Can you work these out from the model? Positions are in its coordinate system, mm. Coordinates: 2 decimals unless noted, no trailing zeros. Write each loop counter-clockwise with the first axis right and the second up, starting at its lowest first coordinate (ties: lowest second). Pieces come first, ordered by that corner, then holes. Notation, with made-up numbers: (-11, -29.5) -> (47, -29.5) arc R8 cw to (47, -17.5) -> close; hole circle Ø4 at (44.25, 72). An arc over 180 degrees is marked (long way). Use one line per item in the form item = value.
Autodesk Inventor part; units mm, degrees
ref_plane "YZ Plane" through (0, 0, 0) normal (1, 0, 0) x (0, 1, 0)
ref_plane "XZ Plane" through (0, 0, 0) normal (0, 1, 0) x (-1, 0, 0)
ref_plane "XY Plane" through (0, 0, 0) normal (0, 0, 1) x (1, 0, 0)
sketch "Sketch3" plane through (0, 0, 0) normal (0, 1, 0) x (-1, 0, 0)
  line L0 (-27.5, -27.5) -> (27.5, -27.5) construction
  line L1 (27.5, -27.5) -> (27.5, 27.5) construction
  line L2 (27.5, 27.5) -> (-27.5, 27.5) construction
  line L3 (-27.5, 27.5) -> (-27.5, -27.5) construction
  line L4 (-27.5, -27.5) -> (27.5, 27.5) construction
  line L5 (27.5, -27.5) -> (-27.5, 27.5) construction
  circle A0 centre (-27.5, 27.5) radius 1.6
  circle A1 centre (27.5, 27.5) radius 1.6
  circle A2 centre (-27.5, -27.5) radius 1.6
  circle A3 centre (27.5, -27.5) radius 1.6
  circle A4 centre (-67.1751, -42.4264) radius 1.6 construction
  line L6 (-27.5, -27.5) -> (-67.1751, -42.4264) construction
  line L7 (-30, -25.7695) -> (-68.0554, -40.0865) construction
  line L8 (-66.2948, -44.7663) -> (-27.0453, -30) construction
  arc A5 (-68.0554, -40.0865) -> (-66.2948, -44.7663) centre (-67.1751, -42.4264) ccw construction
  circle A6 centre (67.1751, -42.4264) radius 1.6 construction
  line L9 (27.5, -27.5) -> (67.1751, -42.4264) construction
  line L10 (27.0453, -30) -> (66.2948, -44.7663) construction
  line L11 (68.0554, -40.0865) -> (30, -25.7695) construction
  arc A7 (66.2948, -44.7663) -> (68.0554, -40.0865) centre (67.1751, -42.4264) ccw construction
  line L12 (27.5, -27.5) -> (-27.5, -27.5) construction
  line L13 (25, -25) -> (-25, -25) construction
  line L14 (-27.0453, -30) -> (27.0453, -30) construction
  line L15 (-27.5, -27.5) -> (-27.5, 27.5) construction
  line L16 (-25, -25) -> (-25, 25) construction
  line L17 (-30, 25.7695) -> (-30, -25.7695) construction
  circle A8 centre (-67.1751, 42.4264) radius 1.6 construction
  line L18 (-27.5, 27.5) -> (-67.1751, 42.4264) construction
  line L19 (-27.0453, 30) -> (-66.2948, 44.7663) construction
  line L20 (-68.0554, 40.0865) -> (-30, 25.7695) construction
  arc A9 (-66.2948, 44.7663) -> (-68.0554, 40.0865) centre (-67.1751, 42.4264) ccw construction
  line L21 (-27.5, 27.5) -> (27.5, 27.5) construction
  line L22 (-25, 25) -> (25, 25) construction
  line L23 (27.0453, 30) -> (-27.0453, 30) construction
  circle A10 centre (67.1751, 42.4264) radius 1.6 construction
  line L24 (27.5, 27.5) -> (67.1751, 42.4264) construction
  line L25 (34.5998, 27.5) -> (68.0554, 40.0865) construction
  line L26 (66.2948, 44.7663) -> (27.0453, 30) construction
  arc A11 (68.0554, 40.0865) -> (66.2948, 44.7663) centre (67.1751, 42.4264) ccw construction
  line L27 (27.5, -27.5) -> (27.5, 27.5) construction
  line L28 (30, -25.7695) -> (30, 25.7695) construction
  line L29 (25, 25) -> (25, -25) construction
  line L30 (34.5998, 27.5) -> (30, 25.7695) construction
  line L31 (55, 55) -> (-55, -55) construction
  line L32 (-55, 55) -> (55, -55) construction
  circle A12 centre (0, 0) radius 110 construction
  arc A13 (43.0581, -98.5) -> (-43.0581, -98.5) centre (0, 0) ccw construction
  line L33 (0, -107.5) -> (0, -98.5) construction
  line L34 (0, -98.5) -> (0, -73.5) construction
  line L35 (0, -98.5) -> (-43.0581, -98.5) construction
  line L36 (0, -98.5) -> (43.0581, -98.5) construction
  line L37 (43.0581, -98.5) -> (-43.0581, -98.5) construction
  line L38 (-18.0581, -73.5) -> (18.0581, -73.5) construction
  arc A14 (43.0581, -98.5) -> (18.0581, -73.5) centre (18.0581, -98.5) ccw construction
  arc A15 (-18.0581, -73.5) -> (-43.0581, -98.5) centre (-18.0581, -98.5) ccw construction
  line L39 (0, 107.5) -> (0, 97.5) construction
  line L40 (0, 97.5) -> (-22.5, 97.5) construction
  line L41 (-22.5, 97.5) -> (-22.5, 82.5) construction
  line L42 (22.5, 82.5) -> (22.5, 97.5) construction
  line L43 (22.5, 90) -> (-22.5, 90) construction
  line L44 (15, 97.5) -> (-15, 97.5)
  line L45 (-15, 82.5) -> (15, 82.5)
  arc A16 (15, 82.5) -> (15, 97.5) centre (15, 90) ccw
  arc A17 (-15, 97.5) -> (-15, 82.5) centre (-15, 90) ccw
  line L46 (22.5, 82.5) -> (17.5, 82.5) construction
  line L47 (17.5, 82.5) -> (17.5, 77.5) construction
  circle A18 centre (17.5, 77.5) radius 1.6
  circle A19 centre (-17.5, 77.5) radius 1.6
  line L48 (-58.3363, 79.5495) -> (-79.5495, 58.3363) construction
  arc A20 (-47.7297, 68.9429) -> (-58.3363, 79.5495) centre (-53.033, 74.2462) ccw construction
  arc A21 (-79.5495, 58.3363) -> (-68.9429, 47.7297) centre (-74.2462, 53.033) ccw construction
  line L49 (-68.9429, 47.7297) -> (-47.7297, 68.9429) construction
  circle A22 centre (-67.1751, 42.4264) radius 1.6 construction
  circle A23 centre (-42.4264, 67.1751) radius 1.6 construction
  line L50 (-97.5, 15) -> (-97.5, -15)
  arc A24 (-82.5, 15) -> (-97.5, 15) centre (-90, 15) ccw
  arc A25 (-97.5, -15) -> (-82.5, -15) centre (-90, -15) ccw
  line L51 (-82.5, -15) -> (-82.5, 15)
  circle A26 centre (-77.5, -17.5) radius 1.6
  circle A27 centre (-77.5, 17.5) radius 1.6
  line L52 (-79.5495, -58.3363) -> (-58.3363, -79.5495) construction
  arc A28 (-68.9429, -47.7297) -> (-79.5495, -58.3363) centre (-74.2462, -53.033) ccw construction
  arc A29 (-58.3363, -79.5495) -> (-47.7297, -68.9429) centre (-53.033, -74.2462) ccw construction
  line L53 (-47.7297, -68.9429) -> (-68.9429, -47.7297) construction
  circle A30 centre (-42.4264, -67.1751) radius 1.6 construction
  circle A31 centre (-67.1751, -42.4264) radius 1.6 construction
  line L54 (-15, -97.5) -> (15, -97.5)
  arc A32 (-15, -82.5) -> (-15, -97.5) centre (-15, -90) ccw
  arc A33 (15, -97.5) -> (15, -82.5) centre (15, -90) ccw
  line L55 (15, -82.5) -> (-15, -82.5)
  circle A34 centre (17.5, -77.5) radius 1.6
  circle A35 centre (-17.5, -77.5) radius 1.6
  line L56 (58.3363, -79.5495) -> (79.5495, -58.3363) construction
  arc A36 (47.7297, -68.9429) -> (58.3363, -79.5495) centre (53.033, -74.2462) ccw construction
  arc A37 (79.5495, -58.3363) -> (68.9429, -47.7297) centre (74.2462, -53.033) ccw construction
  line L57 (68.9429, -47.7297) -> (47.7297, -68.9429) construction
  circle A38 centre (67.1751, -42.4264) radius 1.6 construction
  circle A39 centre (42.4264, -67.1751) radius 1.6 construction
  line L58 (97.5, -15) -> (97.5, 15)
  arc A40 (82.5, -15) -> (97.5, -15) centre (90, -15) ccw
  arc A41 (97.5, 15) -> (82.5, 15) centre (90, 15) ccw
  line L59 (82.5, 15) -> (82.5, -15)
  circle A42 centre (77.5, 17.5) radius 1.6
  circle A43 centre (77.5, -17.5) radius 1.6
  line L60 (79.5495, 58.3363) -> (58.3363, 79.5495) construction
  arc A44 (68.9429, 47.7297) -> (79.5495, 58.3363) centre (74.2462, 53.033) ccw construction
  arc A45 (58.3363, 79.5495) -> (47.7297, 68.9429) centre (53.033, 74.2462) ccw construction
  line L61 (47.7297, 68.9429) -> (68.9429, 47.7297) construction
  circle A46 centre (42.4264, 67.1751) radius 1.6 construction
  circle A47 centre (67.1751, 42.4264) radius 1.6 construction
  line L62 (58.3363, -58.3363) -> (51.2652, -51.2652) construction
  line L63 (40.6586, -61.8718) -> (61.8718, -40.6586) construction
  arc A48 (40.6586, -61.8718) -> (44.5267, -89.5398) centre (53.033, -74.2462) ccw construction
  arc A49 (89.5398, -44.5267) -> (61.8718, -40.6586) centre (74.2462, -53.033) ccw construction
  line L64 (0, -73.5) -> (0, -66.5) construction
  arc A50 (44.5267, 89.5398) -> (40.6586, 61.8718) centre (53.033, 74.2462) ccw construction
  line L65 (61.8718, 40.6586) -> (40.6586, 61.8718) construction
  arc A51 (61.8718, 40.6586) -> (89.5398, 44.5267) centre (74.2462, 53.033) ccw construction
  arc A52 (-89.5398, 44.5267) -> (-61.8718, 40.6586) centre (-74.2462, 53.033) ccw construction
  line L66 (-40.6586, 61.8718) -> (-61.8718, 40.6586) construction
  arc A53 (-40.6586, 61.8718) -> (-44.5267, 89.5398) centre (-53.033, 74.2462) ccw construction
  arc A54 (-44.5267, -89.5398) -> (-40.6586, -61.8718) centre (-53.033, -74.2462) ccw construction
  line L67 (-61.8718, -40.6586) -> (-40.6586, -61.8718) construction
  arc A55 (-61.8718, -40.6586) -> (-89.5398, -44.5267) centre (-74.2462, -53.033) ccw construction
  arc A56 (89.5398, -44.5267) -> (89.5398, 44.5267) centre (0, 0) ccw construction
  arc A57 (44.5267, 89.5398) -> (-44.5267, 89.5398) centre (0, 0) ccw construction
  arc A58 (-89.5398, 44.5267) -> (-89.5398, -44.5267) centre (0, 0) ccw construction
  line L68 (43.0581, -98.5) -> (48.0581, -98.5) construction
  line L69 (48.0581, -98.5) -> (48.0581, -88.5) construction
  circle A59 centre (48.0581, -88.5) radius 1.6 construction
  circle A60 centre (-48.0581, -88.5) radius 1.6 construction
  line L70 (18.0581, -66.5) -> (-18.0581, -66.5) construction
  arc A61 (17.5, -66.5) -> (43.0581, -59.4724) centre (19.5145, -23.8377) ccw construction
  arc A62 (-44.5267, -58.0038) -> (-18.0581, -66.5) centre (-19.5089, -25.5422) ccw construction
  line L71 (0, -66.5) -> (0, -41.5) construction
  line L72 (0, -41.5) -> (50, -41.5)
  line L73 (0, -41.5) -> (-50, -41.5)
  line L74 (107.5, 0) -> (70, 0) construction
  line L75 (70, 0) -> (70, -30)
  line L76 (70, 0) -> (70, 30)
  line L77 (-70, 0) -> (-70, -30)
  line L78 (-70, 0) -> (-70, 30)
  arc A63 (70, -30) -> (50, -41.5) centre (69.3076, -51.9372) ccw
  arc A64 (-50, -41.5) -> (-70, -30) centre (-72.2179, -56.9986) ccw
  line L79 (0, 0) -> (15.9, 0) construction
  line L80 (0, 41.5) -> (50, 41.5)
  line L81 (0, 41.5) -> (-50, 41.5)
  arc A65 (50, 41.5) -> (70, 30) centre (69.3076, 51.9372) ccw
  arc A66 (-70, 30) -> (-50, 41.5) centre (-72.2179, 56.9986) ccw
  point P0 (-47.3376, -34.9632)
  point P1 (47.3376, -34.9632)
  point P2 (0, -27.5)
  point P3 (-27.5, 0)
  point P4 (-47.3376, 34.9632)
  point P5 (0, 27.5)
  point P6 (47.3376, 34.9632)
  point P7 (27.5, 0)
  point P8 (0, 90)
  point P9 (-45.9619, 70.7107)
  point P10 (-82.5, 17.5)
  point P11 (-70.7107, -45.9619)
  point P12 (-17.5, -82.5)
  point P13 (45.9619, -70.7107)
  point P14 (82.5, -17.5)
  point P15 (70.7107, 45.9619)
  point P16 (35.7159, -76.7698)
  dimension "d50" = 55
  dimension "d51" = 55
  dimension "d52" = 3.2
  dimension "d53" = 3.2
  dimension "d54" = 3.2
  dimension "d55" = 3.2
  dimension "d56" = 5
  dimension "d57" = 5
  dimension "d58" = 5
  dimension "d59" = 5
  dimension "d60" = 110
  dimension "d67" = 220
  dimension "d68" = 215
  dimension "d69" = 9
  dimension "d70" = 25
  dimension "d71" = 10
  dimension "d72" = 22.5
  dimension "d73" = 15
  dimension "d74" = 45
  dimension "d75" = 5
  dimension "d76" = 5
  dimension "d77" = 3.2
  dimension "d78" = 86.1162
  dimension "d79" = 45
  dimension "d80" = 360
  dimension "d81" = 10
  dimension "d82" = 7
  dimension "d83" = 360
  dimension "d84" = 5
  dimension "d85" = 10
  dimension "d86" = 3.2
  dimension "d87" = 25
  dimension "d88" = 50
  dimension "d89" = 50
  dimension "d90" = 37.5
  dimension "d91" = 30
  dimension "d92" = 30
extrude "Extrusion3" add sketch "Sketch3" along normal blind 1 contours L73 A64 L77 L78 A66 L81 L80 A65 L76 L75 A63 L72
fillet "Fillet1" radius 2 8 edges at (50, 0.5, 41.5) (70, 0.5, 30) (70, 0.5, -30) (50, 0.5, -41.5) (-50, 0.5, 41.5) (-70, 0.5, 30) (-70, 0.5, -30) (-50, 0.5, -41.5)
properties part number "Infrared&ControllerPCB" material "Aluminum 6061"
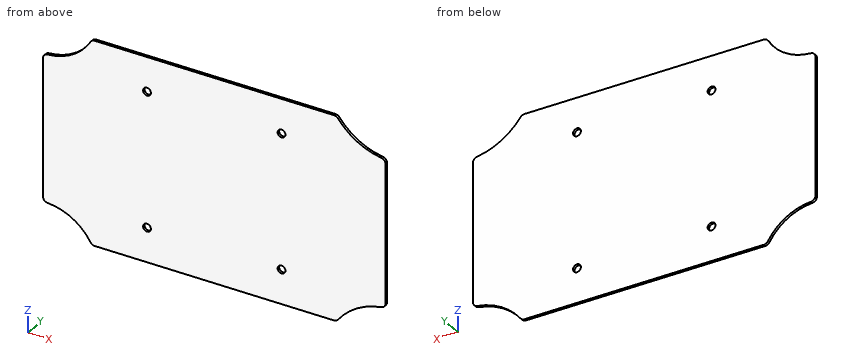
Q1. Suppose I cut it at A-A (x = 27.5). Write out the boundary of the cut face in (y, z), then the cut area to 3 significant figures.
Return value:
outline = (0, -41.5) -> (1, -41.5) -> (1, -29.1) -> (0, -29.1) -> close; (0, -25.9) -> (1, -25.9) -> (1, 25.9) -> (0, 25.9) -> close; (0, 29.1) -> (1, 29.1) -> (1, 41.5) -> (0, 41.5) -> close
area = 76.6 mm2
Q2. Will this pin go through, and if not, where does the flat tip stop? pin 1 (2.5 mm diameter, centred on x = 27.5, z = -27.5, fed in from +Y).
Return value:
pin_1 = through
Q3. If I drill on line 1 (Z direction, x = -27.5, y = 0.75); line 2 (Z direction, x = -27, y = 0.45); line 3 (Z direction, x = -63, y = 0.4) (3 decimals), over which ranges is the centre line in solid material (lowest first)? Write a range as from..to.
Return value:
line_1 = -41.5..-29.1, -25.9..25.9, 29.1..41.5
line_2 = -41.5..-29.02, -25.98..25.98, 29.02..41.5
line_3 = -30.915..30.915
Q4. Suppose I cut it at C-C (z = 34.5). Write out the boundary of the cut face in (x, y), then the cut area to 3 significant figures.
Return value:
outline = (-55.98, 0) -> (57.13, 0) -> (57.13, 1) -> (-55.98, 1) -> close
area = 113 mm2
Q5. Suppose I cut it at B-B (y = 0.15). Write out the boundary of the cut face in (x, z), then the cut area to 3 significant figures.
Return value:
outline = (-70, -28.02) arc R2 ccw to (-68.11, -30.02) arc R21.95 cw to (-50.55, -40.54) arc R2 ccw to (-48.84, -41.5) -> (48.98, -41.5) arc R2 ccw to (50.58, -40.7) arc R27.09 cw to (68.29, -30.2) arc R2 ccw to (70, -28.22) -> (70, 28.22) arc R2 ccw to (68.29, 30.2) arc R27.09 cw to (50.58, 40.7) arc R2 ccw to (48.98, 41.5) -> (-48.84, 41.5) arc R2 ccw to (-50.55, 40.54) arc R21.95 cw to (-68.11, 30.02) arc R2 ccw to (-70, 28.02) -> close; hole circle Ø3.2 at (-27.5, -27.5); hole circle Ø3.2 at (-27.5, 27.5); hole circle Ø3.2 at (27.5, -27.5); hole circle Ø3.2 at (27.5, 27.5)
area = 10,900 mm2
